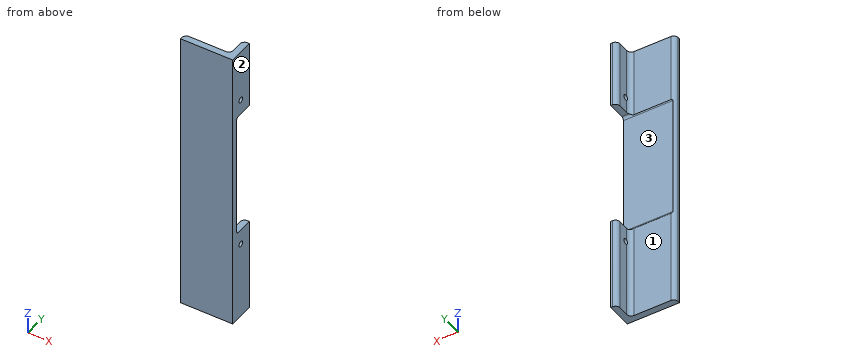
from build123d import *

# Parameters (mm, degrees)
F1_DEPTH = 139.7
F2_R     = 1.3462
F3_DEPTH = 25.2994
F5_DEPTH = 25.2994


with BuildPart() as f1:
    # F0 (on Top) → F1 (new body)
    with BuildSketch(Plane.XY):
        with BuildLine():
            Line((-15.458836, -4.64103), (-15.458836, -5.60623))
            Line((-15.458836, -5.60623), (9.839564, -5.60623))
            Line((9.839564, -5.60623), (9.839564, 6.99217))
            Line((9.839564, 6.99217), (8.874364, 6.99217))
            ThreePointArc((8.874364, 6.99217), (7.34772, 6.359813), (6.715364, 4.83317))
            Line((6.715364, 4.83317), (6.715364, -0.32303))
            ThreePointArc((6.715364, -0.32303), (6.083007, -1.849674), (4.556364, -2.48203))
            Line((4.556364, -2.48203), (-13.299836, -2.48203))
            ThreePointArc((-13.299836, -2.48203), (-14.82648, -3.114387), (-15.458836, -4.64103))
        make_face()
    extrude(amount=F1_DEPTH)

    # F2 (on face) → F3 (cut, through all)
    with BuildSketch(Plane.YZ.offset(9.839564)):
        with Locations((0.48977, 38.1)):
            Circle(F2_R)
        with Locations((0.48977, 114.3)):
            Circle(F2_R)
    extrude(amount=-F3_DEPTH, mode=Mode.SUBTRACT)

    # F4 (on face) → F5 (cut, through all)
    with BuildSketch(Plane.YZ.offset(9.839564)):
        with BuildLine():
            Line((-1.41523, 45.5422), (6.99217, 45.5422))
            Line((6.99217, 45.5422), (6.99217, 106.8578))
            Line((6.99217, 106.8578), (-1.41523, 106.8578))
            ThreePointArc((-1.41523, 106.8578), (-2.313256, 106.485826), (-2.68523, 105.5878))
            Line((-2.68523, 105.5878), (-2.68523, 46.8122))
            ThreePointArc((-2.68523, 46.8122), (-2.313256, 45.914174), (-1.41523, 45.5422))
        make_face()
    extrude(amount=-F5_DEPTH, mode=Mode.SUBTRACT)


solid = f1.part
Here's how the part is built. I have some questions about the finished solid (model axes, mm). Face numbers are marked on the shaded views. A direction names the side the tool comes from. Round coordinates to 2 decimals unless told otherwise and drop trailing zeros. Loops run counter-clockwise (first coordinate to the right, second up) from the corner with the lowest first, then second, coordinate; pieces in that order, holes last.
1. If we section it at A-A on z = 130.5: Write out the boundary of the cut face in (x, y), plus the area to 3 significant figures.
Answer list:
outline: (-15.46, -5.61) - (9.84, -5.61) - (9.84, 6.99) - (8.87, 6.99) arc R2.16 ccw to (6.72, 4.83) - (6.72, -0.32) arc R2.16 cw to (4.56, -2.48) - (-13.3, -2.48) arc R2.16 ccw to (-15.46, -4.64) - close
area: 108 mm2
2. For P1, Ø5, axis at y = 0.5, z = 26, coming from the -X side; P2, Ø4, axis at y = 1, z = 122.5, coming from the -X side; P3, Ø5.5, axis at y = 1, z = 28.5, coming from the -X side, each with a flat end and sliding along its axis, tell me the tip position at first contact or that it passes through.
Answer list:
P1: stops at x = 5.92
P2: stops at x = 6.61
P3: stops at x = 6.18
3. If we section it at B-B on x = -8.75: Write out the boundary of the cut face in (y, z), plus the area to 3 significant figures.
Answer list:
outline: (-5.61, 0) - (-2.48, 0) - (-2.48, 46.12) arc R1.27 cw to (-2.69, 46.81) - (-2.69, 105.59) arc R1.27 cw to (-2.48, 106.28) - (-2.48, 139.7) - (-5.61, 139.7) - close
area: 424 mm2
4. If we section it at C-C on z = 59: Write out the boundary of the cut face in (x, y), plus the area to 3 significant figures.
Answer list:
outline: (-15.46, -5.61) - (9.84, -5.61) - (9.84, -2.69) - (-14.21, -2.69) arc R2.16 ccw to (-15.46, -4.64) - close
area: 73.2 mm2
5. If I drill on line 1 along Y through (x, z) = (9.15, 38.1); line 2 along Y through (x, z) = (8.5, 98); line 3 along Y through (x, z) = (-12.25, 37.5), over which ranges is the centre line in solid material (lowest first)?
Answer list:
line 1: y = -5.61 to -0.86, 1.84 to 6.99
line 2: y = -5.61 to -2.69
line 3: y = -5.61 to -2.48
6. Which directions (+Z, -Z, +X, -X, +Y, -Y) give clear straight access to the entire face, cutting with the end or side of a thin tool? Please do the marked faces 1, 2 and 3.
Answer list:
face 1: +Z, -Z, -X, +Y
face 2: +Z, -Z, +X, +Y, -Y
face 3: +X, -X, +Y
